from build123d import *

# Parameters (mm, degrees)
F0_W      = 7
F0_H      = 7
F0_W_2    = 3
F0_H_2    = 5
F0_W_3    = 6
F0_H_3    = 11
F1_DEPTH  = 3
F2_DEPTH  = 6
F3_W      = 3
F3_H      = 1.5
F4_DEPTH  = 2
F5_W      = 3
F5_H      = 1.5
F6_DEPTH  = 2
F7_W      = 2.4
F7_H      = 1.5
F8_DEPTH  = 6
F10_DEPTH = 7
F11_R     = 1.435
F12_DEPTH = 4
F14_DEPTH = 5
F15_DEPTH = 5
F16_DEPTH = 5
F17_DEPTH = 5


with BuildPart() as f1:
    # F0 (on Top) → F1 (new body)
    with BuildSketch(Plane.XY):
        Polygon((40, 11.75), (-40, 11.75), (-40, -3.75), (-33, -3.75), (-33, -11.75), (33, -11.75), (33, -3.75), (40, -3.75), align=None)
        with Locations((-33.5, 3.25)):
            Rectangle(F0_W, F0_H, mode=Mode.SUBTRACT)
        with Locations((-18.002523, 6.25)):
            Rectangle(F0_W_2, F0_H_2, mode=Mode.SUBTRACT)
        with Locations((0, 2.75)):
            Rectangle(F0_W_3, F0_H_3, mode=Mode.SUBTRACT)
        with Locations((33.5, 3.25)):
            Rectangle(F0_W, F0_H, mode=Mode.SUBTRACT)
        with Locations((18.002523, 6.25)):
            Rectangle(F0_W_2, F0_H_2, mode=Mode.SUBTRACT)
    extrude(amount=F1_DEPTH)

    # F0 (on Top) → F2 (join)
    with BuildSketch(Plane.XY):
        with Locations((-18.002523, 6.25)):
            Rectangle(F0_W_2, F0_H_2)
        with Locations((18.002523, 6.25)):
            Rectangle(F0_W_2, F0_H_2)
    extrude(amount=F2_DEPTH)

    # F3 (on face) → F4 (cut)
    with BuildSketch(Plane(origin=(0, 8.75, 0), x_dir=(-1, 0, 0), z_dir=(0, 1, 0))):
        with Locations((-18.002523, 3.75)):
            Rectangle(F3_W, F3_H)
    extrude(amount=-F4_DEPTH, mode=Mode.SUBTRACT)

    # F5 (on face) → F6 (cut)
    with BuildSketch(Plane(origin=(0, 8.75, 0), x_dir=(-1, 0, 0), z_dir=(0, 1, 0))):
        with Locations((18.002523, 3.75)):
            Rectangle(F5_W, F5_H)
    extrude(amount=-F6_DEPTH, mode=Mode.SUBTRACT)

    # F7 (on face) → F8 (join)
    with BuildSketch(Plane(origin=(0, 11.75, 0), x_dir=(-1, 0, 0), z_dir=(0, 1, 0))):
        with Locations((0, 0.75)):
            Rectangle(F7_W, F7_H)
    extrude(amount=F8_DEPTH)

    # F9 (on face) → F10 (join)
    with BuildSketch(Plane.XZ.offset(11.75)):
        with BuildLine():
            Line((-30, 3), (-24, 3))
            ThreePointArc((-24, 3), (-27, 6), (-30, 3))
        make_face()
        with BuildLine():
            ThreePointArc((-16, 3), (-19, 6), (-22, 3))
            Line((-22, 3), (-16, 3))
        make_face()
        with BuildLine():
            ThreePointArc((22, 3), (19, 6), (16, 3))
            Line((16, 3), (22, 3))
        make_face()
        with BuildLine():
            ThreePointArc((30, 3), (27, 6), (24, 3))
            Line((24, 3), (30, 3))
        make_face()
    extrude(amount=-F10_DEPTH)

    # F11 (on face) → F12 (cut)
    with BuildSketch(Plane.XZ.offset(11.75)):
        with Locations((-27, 3)):
            Circle(F11_R)
        with Locations((-19, 3)):
            Circle(F11_R)
        with Locations((19, 3)):
            Circle(F11_R)
        with Locations((27, 3)):
            Circle(F11_R)
    extrude(amount=-F12_DEPTH, mode=Mode.SUBTRACT)

    # F13 (on face) → F14 (join)
    with BuildSketch(Plane(origin=(0, 11.75, 0), x_dir=(-1, 0, 0), z_dir=(0, 1, 0))):
        with BuildLine():
            Line((-30.125, 3), (-30.125, 4.15))
            ThreePointArc((-30.125, 4.15), (-33.508255, 7.52499), (-36.87496, 4.133489))
            Line((-36.87496, 4.133489), (-36.87496, 3))
            Line((-36.87496, 3), (-34.576162, 3))
            ThreePointArc((-34.576162, 3), (-34.126765, 5.594919), (-31.925, 4.15))
            ThreePointArc((-31.925, 4.15), (-32.055081, 3.523235), (-32.423838, 3))
            Line((-32.423838, 3), (-30.125, 3))
        make_face()
        with BuildLine():
            Line((-34.576162, 3), (-32.423838, 3))
            ThreePointArc((-32.423838, 3), (-32.055081, 3.523235), (-31.925, 4.15))
            ThreePointArc((-31.925, 4.15), (-34.126765, 5.594919), (-34.576162, 3))
        make_face()
    extrude(amount=-F14_DEPTH)

    # F13 (on face) → F15 (cut, through all)
    with BuildSketch(Plane(origin=(0, 11.75, 0), x_dir=(-1, 0, 0), z_dir=(0, 1, 0))):
        with BuildLine():
            Line((-34.576162, 3), (-32.423838, 3))
            ThreePointArc((-32.423838, 3), (-32.055081, 3.523235), (-31.925, 4.15))
            ThreePointArc((-31.925, 4.15), (-34.126765, 5.594919), (-34.576162, 3))
        make_face()
        with BuildLine():
            ThreePointArc((-34.576162, 3), (-33.5, 2.575), (-32.423838, 3))
            Line((-32.423838, 3), (-34.576162, 3))
        make_face()
    extrude(amount=-F15_DEPTH, mode=Mode.SUBTRACT)

    # F13 (on face) → F16 (join)
    with BuildSketch(Plane(origin=(0, 11.75, 0), x_dir=(-1, 0, 0), z_dir=(0, 1, 0))):
        with BuildLine():
            Line((30.125, 4.15), (30.125, 3))
            Line((30.125, 3), (32.423838, 3))
            ThreePointArc((32.423838, 3), (32.873235, 5.594919), (35.075, 4.15))
            ThreePointArc((35.075, 4.15), (34.944919, 3.523235), (34.576162, 3))
            Line((34.576162, 3), (36.87496, 3))
            Line((36.87496, 3), (36.87496, 4.133489))
            ThreePointArc((36.87496, 4.133489), (33.508255, 7.52499), (30.125, 4.15))
        make_face()
        with BuildLine():
            Line((34.576162, 3), (32.423838, 3))
            ThreePointArc((32.423838, 3), (33.5, 2.575), (34.576162, 3))
        make_face()
        with BuildLine():
            ThreePointArc((35.075, 4.15), (32.873235, 5.594919), (32.423838, 3))
            Line((32.423838, 3), (34.576162, 3))
            ThreePointArc((34.576162, 3), (34.944919, 3.523235), (35.075, 4.15))
        make_face()
    extrude(amount=-F16_DEPTH)

    # F13 (on face) → F17 (cut, through all)
    with BuildSketch(Plane(origin=(0, 11.75, 0), x_dir=(-1, 0, 0), z_dir=(0, 1, 0))):
        with BuildLine():
            ThreePointArc((35.075, 4.15), (32.873235, 5.594919), (32.423838, 3))
            Line((32.423838, 3), (34.576162, 3))
            ThreePointArc((34.576162, 3), (34.944919, 3.523235), (35.075, 4.15))
        make_face()
        with BuildLine():
            Line((34.576162, 3), (32.423838, 3))
            ThreePointArc((32.423838, 3), (33.5, 2.575), (34.576162, 3))
        make_face()
    extrude(amount=-F17_DEPTH, mode=Mode.SUBTRACT)


solid = f1.part
For this review, take the finished solid that the model builds, in its own axes (mm). A direction names the side the tool comes from. Coordinates: 2 decimals unless noted, no trailing zeros. Order: outer loops, then holes, each group sorted by start corner. A loop starts at its lowest first (then second) coordinate and runs counter-clockwise, first axis right, second up. Notation, with made-up numbers: (47, -3) - (85, -3) arc R23 ccw to (85, 13) - close; hole circle Ø11 at (24, 33.25). An arc over 180 degrees is marked (long way). Use one line per item in the form item = value.
Q1. Consider section B-B (x = 27). Give the boundary of the cut face in (y, z) (3 decimals), then the cut area to 3 significant figures.
Checked values:
outline = (-11.75, 0) - (11.75, 0) - (11.75, 3) - (-4.75, 3) - (-4.75, 6) - (-11.75, 6) - (-11.75, 4.435) - (-7.75, 4.435) - (-7.75, 1.565) - (-11.75, 1.565) - close
area = 80.0 mm2
Q2. For faces 1 (the cylindrical face through (-25.674, -9.778, 2.45)), 2 (the flat face through (18, 8, 4.5)), 3 (the flat face through (33, 6.75, 2)), 4 (the flat face through (18, 8.75, 5)), 5 (the flat face through (-18, 3.75, 4)), list the 3-axis set-ups (+Z, -Z, +X, -X, +Y, -Y) from which the entire face can be reached by the end or side of a thin tool; tool diameter is ignored.
Checked values:
face_1 = -Y
face_2 = +Y
face_3 = +Z, -Z
face_4 = +Z, +Y
face_5 = +Z, +X, -X
Q3. For P1, Ø3.5, axis at x = -34, z = 2, coming from the +Y side; P2, Ø2, axis at y = 14.5, z = 1.5, coming from the +X side; P3, Ø1.5, axis at x = -27.5, z = 4, coming from the +Y side, all flat-tipped, find the tip position at first contact; note any pin that passes through.
Checked values:
P1 = 11.75
P2 = 1.2
P3 = -4.75
Q4. Draft analysis for pull direction X (two halves, no side actions). For faces 6 (the flat face through (-37, 3, 1)), 7 (the flat face through (-27, -4.75, 4)), state which applies: +X half, -X half, draft (parallel to the pull), parting line (faces both ways), or undercut.
Checked values:
face_6 = undercut
face_7 = draft
Q5. Consider section D-D (y = 13.5). Give the boundary of the cut face in (x, z).
Checked values:
outline = (-1.2, 0) - (1.2, 0) - (1.2, 1.5) - (-1.2, 1.5) - close
Q6. Consider section C-C (y = -1). Give the boundary of the cut face in (x, z).
Checked values:
outline = (-40, 0) - (-3, 0) - (-3, 3) - (-40, 3) - close; (3, 0) - (40, 0) - (40, 3) - (3, 3) - close
Q7. Consider section A-A (y = 4.5). Give the boundary of the cut face in (x, z).
Checked values:
outline = (-40, 0) - (-37, 0) - (-37, 3) - (-40, 3) - close; (-30, 0) - (-3, 0) - (-3, 3) - (-16.5, 3) - (-16.5, 6) - (-19.5, 6) - (-19.5, 3) - (-30, 3) - close; (3, 0) - (30, 0) - (30, 3) - (19.5, 3) - (19.5, 6) - (16.5, 6) - (16.5, 3) - (3, 3) - close; (37, 0) - (40, 0) - (40, 3) - (37, 3) - close
Q8. For probe 1 along X at (y, z) = (10.2, 4.15) (3 decimals); probe 2 along X at (y, z) = (6.5, 1.25); probe 3 along Y at (x, z) = (31, 0.5), list the stretches that pass through material, from the lowest coordinate up. Write a range as from..to.
Checked values:
probe_1 = -36.875..-35.075, -31.925..-30.125, 30.125..31.925, 35.075..36.875
probe_2 = -40..-37, -30..-3, 3..30, 37..40
probe_3 = -11.75..-0.25, 6.75..11.75
